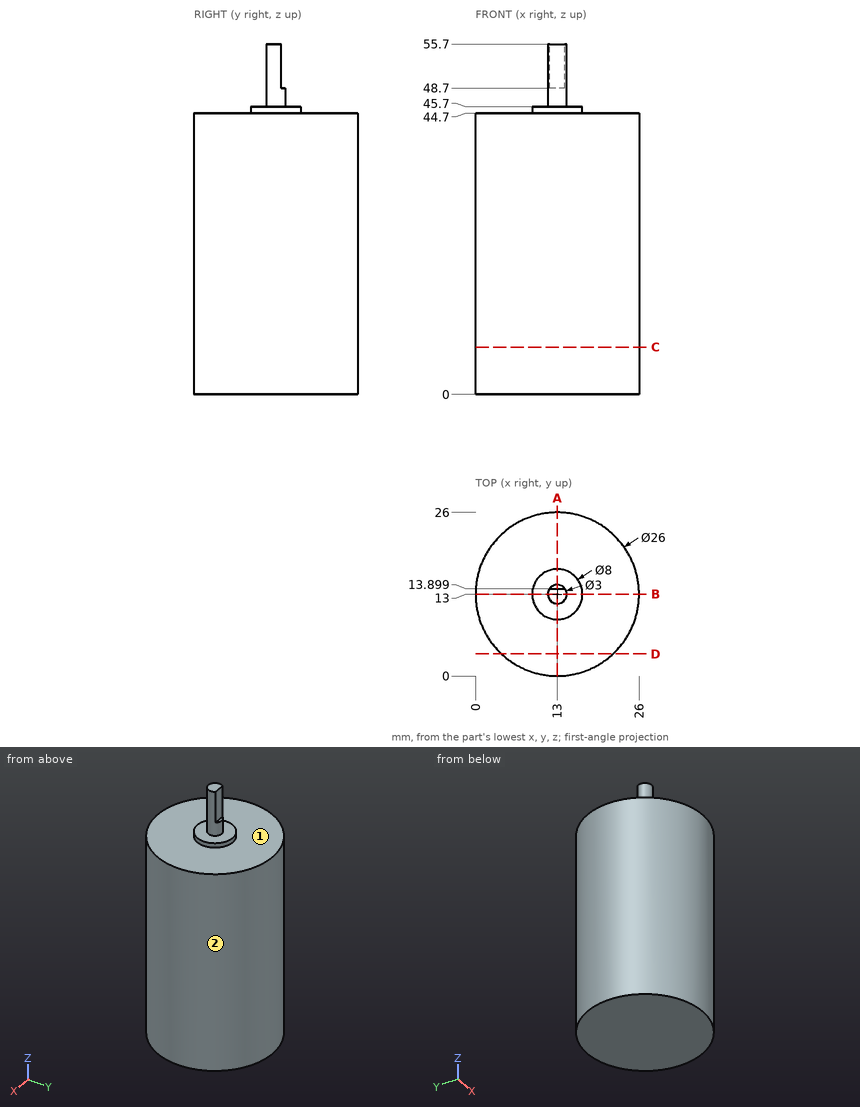
Geometry: see drawing. Coordinates: mm, zero at the bounding-box minimum. A direction names the side the tool comes from. Give positions to 0.01 mm unless a question says otherwise; leave off trailing zeros. Order: outer loops, then holes, each group sorted by start corner. A loop starts at its lowest first (then second) coordinate and runs counter-clockwise, first axis right, second up. Notation, with made-up numbers: M 52.25,49 L 96.25,49 A5 ccw 96.25,53 Z; hole C 39,-14.5 d4. An arc over 180 degrees is marked long. Answer as CSV lines item,"result". Start each with the question number.
1) Cut plane C-C (z = 7.5). Output: boundary loops of the cut face in (x, y).
2) Cut plane A-A (x = 13). Output: boundary loops of the cut face in (y, z), then the cut area to 3 significant figures.
3) First-contact query: P1, Ø0.7, axis at x = 13, z = 51, coming from the +Y side; P2, Ø3, axis at y = 19, z = 43.5, coming from the -X side; P3, Ø6, axis at y = 23, z = 17.5, coming from the +X side (1 decimal). Flat tips, straight axial feed; report the tip coordinate or a pass-through.
4) Line query: line 1 (Z direction, x = 24.25, y = 9.5); line 2 (Y direction, x = 12.5, z = 6); line 3 (Z direction, x = 10.25, y = 13.75). Output: solid intervals per line, ascending. Write a range as from..to.
5) Set-up query: the marked faces 1 and 2. Return all of +Z, -Z, +X, -X, +Y, -Y with unobstructed straight access to the full face (end or side cutting, diameter ignored); none if empty.
6) Cut plane B-B (y = 13). Output: boundary loops of the cut face in (x, z), then the cut area to 3 significant figures.
7) Cut plane D-D (y = 3.5). Output: boundary loops of the cut face in (x, z).
Findings below:
1,outline,"C 13,13 d26"
2,outline,"M 0,0 L 26,0 L 26,44.7 L 17,44.7 L 17,45.7 L 14.5,45.7 L 14.5,48.7 L 13.9,48.7 L 13.9,55.7 L 11.5,55.7 L 11.5,45.7 L 9,45.7 L 9,44.7 L 0,44.7 Z"
2,area,"1,200 mm²"
3,P1,"stops at y = 13.9"
3,P2,"stops at x = 0.8"
3,P3,"stops at x = 24"
4,line 1,"z = 0..44.7"
4,line 2,"y = 0.01..25.99"
4,line 3,"z = 0..45.7"
5,face 1,"+Z"
5,face 2,"+Z, -Z"
6,outline,"M 0,0 L 26,0 L 26,44.7 L 17,44.7 L 17,45.7 L 14.5,45.7 L 14.5,55.7 L 11.5,55.7 L 11.5,45.7 L 9,45.7 L 9,44.7 L 0,44.7 Z"
6,area,"1,200 mm²"
7,outline,"M 4.13,0 L 21.87,0 L 21.87,44.7 L 4.13,44.7 Z"
